Read the model definition and answer for the solid it produces. Units are mm, in the model's axes. A direction names the side the tool comes from. Give positions to 0.01 mm unless a question says otherwise; leave off trailing zeros. Write each loop counter-clockwise with the first axis right and the second up, starting at its lowest first coordinate (ties: lowest second). Pieces come first, ordered by that corner, then holes. Notation, with made-up numbers: (-38, 45.5) -> (4, 45.5) arc R29 cw to (4, 65.5) -> close; hole circle Ø5 at (73.5, -35.75). An arc over 180 degrees is marked (long way). Use a Markdown table: item, result.
from build123d import *

# Parameters (mm, degrees)
EXTRUDE_1_DEPTH     = 3
SKETCH_2_R          = 2.4
EXTRUDE_2_DEPTH     = 10
EXTRUDE_3_DEPTH     = 3
SKETCH_4_R          = 1.65
CUT_EXTRUDE_1_DEPTH = 26.475478406


with BuildPart() as part:
    # 草图1 → 凸台-拉伸1 (new body)
    with BuildSketch(Plane(origin=(0, 0, 0), x_dir=(1, 0, 0), z_dir=(0, 1, 0))):
        with BuildLine():
            Line((0, 7.5), (18, 7.5))
            Line((18, 7.5), (18, -7.5))
            Line((18, -7.5), (0, -7.5))
            ThreePointArc((0, -7.5), (-7.5, 0), (0, 7.5))
        make_face()
    extrude(amount=EXTRUDE_1_DEPTH)

    # 草图2 → 凸台-拉伸2 (add)
    with BuildSketch(Plane.XZ):
        with Locations(Location((0, 0, 0), (0, 0, 90))):
            Circle(SKETCH_2_R)
    extrude(amount=EXTRUDE_2_DEPTH)

    # 草图3 → 凸台-拉伸3 (add)
    with BuildSketch(Plane.XY.offset(7.5)):
        Polygon((18, 3), (8, 3), (10, 9), (16, 9), align=None)
    extrude_3 = extrude(amount=-EXTRUDE_3_DEPTH)

    # 镜向1: 凸台-拉伸3 across plane
    add(extrude_3.mirror(Plane.XY))

    # 草图4 → 切除-拉伸1 (cut, through all)
    with BuildSketch(Plane.XY.offset(7.5)):
        with Locations((13, 5.5)):
            Circle(SKETCH_4_R)
    extrude(amount=-CUT_EXTRUDE_1_DEPTH, mode=Mode.SUBTRACT)


solid = part.part
Item 1: For a pull along Y with two mould halves and no side action, classify faces 4 (the face through (0, -10, 0)), 5 (the face through (13, 9, 6)), 6 (the face through (14.524, 4.868, -5.979)), 7 (the face through (14, 7, -4.5)) as +Y half, -Y half, draft (parallel to the pull), parting line (faces both ways), or undercut.
Return value:
| item | result |
|---|---|
| face 4 | -Y half |
| face 5 | +Y half |
| face 6 | undercut |
| face 7 | draft |
Item 2: Each of these flat-tipped pins is pushed along its axis until it touches: P1, Ø2, axis at x = -2, z = 4.5, coming from the -Y side; P2, Ø1.5, axis at y = 2.5, z = 4, coming from the -X side; P3, Ø6, axis at x = 2.5, z = -2.5, coming from the +Y side. Where does it stop, or does it pass through?
Return value:
| item | result |
|---|---|
| P1 | y = 0 |
| P2 | x = -6.76 |
| P3 | y = 3 |
Item 3: A cutting plane is placed at C-C (y = 8). Give the vertices of the cut face in (x, z).
Return value:
| item | result |
|---|---|
| outline | (9.67, -7.5) -> (16.33, -7.5) -> (16.33, -4.5) -> (9.67, -4.5) -> close; (9.67, 4.5) -> (16.33, 4.5) -> (16.33, 7.5) -> (9.67, 7.5) -> close |
Item 4: Straight lines are drawn through the part: line 1 along Y through (x, z) = (13, 6.2); line 2 along Y through (x, z) = (-2.5, -2.5); line 3 along X through (y, z) = (6.5, 5.5). For each, find the intervals that lie inside material, in ascending order. Write a range as [from, to].
Return value:
| item | result |
|---|---|
| line 1 | [0, 3.85], [7.15, 9] |
| line 2 | [0, 3] |
| line 3 | [9.17, 11.69], [14.31, 16.83] |
Item 5: A tool of negligible diameter and unlimited length cuts with its end or side. For faces 1 (the face through (14, 7, 4.5)), 2 (the face through (5, 3, 0)), 3 (the face through (-2.024, -4.93, 1.29)), from which of +Z, -Z, +X, -X, +Y, -Y can it reach the whole face along a straight path? Write none if from no direction.
Return value:
| item | result |
|---|---|
| face 1 | +X, -X, +Y |
| face 2 | -X, +Y |
| face 3 | -Y |
Item 6: A cutting plane is placed at A-A (x = 13). Give the vertices of the cut face in (y, z), then the cut area to 3 significant figures.
Return value:
| item | result |
|---|---|
| outline | (0, -7.5) -> (3.85, -7.5) -> (3.85, -4.5) -> (3, -4.5) -> (3, 4.5) -> (3.85, 4.5) -> (3.85, 7.5) -> (0, 7.5) -> close; (7.15, -7.5) -> (9, -7.5) -> (9, -4.5) -> (7.15, -4.5) -> close; (7.15, 4.5) -> (9, 4.5) -> (9, 7.5) -> (7.15, 7.5) -> close |
| area | 61.2 mm^2 |
Item 7: A cutting plane is placed at D-D (y = 5.5). Give the vertices of the cut face in (x, z), then the cut area to 3 significant figures.
Return value:
| item | result |
|---|---|
| outline | (8.83, -7.5) -> (11.35, -7.5) -> (11.35, -4.5) -> (8.83, -4.5) -> close; (8.83, 4.5) -> (11.35, 4.5) -> (11.35, 7.5) -> (8.83, 7.5) -> close; (14.65, -7.5) -> (17.17, -7.5) -> (17.17, -4.5) -> (14.65, -4.5) -> close; (14.65, 4.5) -> (17.17, 4.5) -> (17.17, 7.5) -> (14.65, 7.5) -> close |
| area | 30.2 mm^2 |
Item 8: A cutting plane is placed at B-B (z = 0). Give the vertices of the cut face in (x, y).
Return value:
| item | result |
|---|---|
| outline | (-7.5, 0) -> (-2.4, 0) -> (-2.4, -10) -> (2.4, -10) -> (2.4, 0) -> (18, 0) -> (18, 3) -> (-7.5, 3) -> close |
